Check sheet for the modelled part. Datum: model origin and axes. Units: mm. A direction names the side the tool comes from. Round coordinates to 2 decimals unless told otherwise and drop trailing zeros. Order: outer loops, then holes, each group sorted by start corner. A loop starts at its lowest first (then second) coordinate and runs counter-clockwise, first axis right, second up.
(1) Sectioned sample at D-D, the plane x = 60. Enter the section's corners in (y, z), and give its area (3 significant figures).
(2) Sectioned sample at B-B, the plane z = 17.5. Enter the section's corners in (x, y), and give its area (3 significant figures).
(3) Tool access check on faces 4 (the flat face through (-57.759, 1.568, 41.056)), 5 (the cylindrical face through (-334.68, 1.57, -7.91)), 6 (the flat face through (68.784, 1.568, -0.502)). Record the directions out of +Z, -Z, +X, -X, +Y, -Y that give a thin tool (end or side, any length) a straight path to the whole face; none if there is none.
(4) Sectioned sample at A-A, the plane y = 1.45. Count the separate pieces of the cut face and the enclosed holes in it, and give its area (3 significant figures).
(5) Mould release check, pull along X, two halves, no side actions. Record for faces 1 (the flat face through (5, 0, 20)), 2 (the flat face through (-70.484, 1.568, 0.147)), 3 (the cylindrical face through (226.448, 1.568, 32.697)): released by +X, released by -X, zero draft, split by the parting line, or undercut.
(6) Sectioned sample at C-C, the plane x = 239. Enter the section's corners in (y, z), and give its area (3 significant figures).
(7) Thickness scan on probe 1 along Z at (x, y) = (0, 2.35); probe 2 along Z at (x, y) = (-325, 1.45) (3 decimals); probe 3 along Z at (x, y) = (-229, 2.4). Record the ranges inside material, lowest first.
```python
from build123d import *

# Parameters (mm, degrees)
BOSS_EXTRUDE1_DEPTH = 3.18
SKETCH3_R           = 3.175
SKETCH3_R_2         = 6.35
SKETCH3_R_3         = 1.65
CUT_EXTRUDE1_DEPTH  = 4.18


with BuildPart() as part:
    # Sketch1 → Boss-Extrude1 (new body)
    with BuildSketch(Plane(origin=(0, 0, 0), x_dir=(1, 0, 0), z_dir=(0, 1, 0))):
        with BuildLine():
            Line((-316.883271773, 9.506246519), (-316.457354569, 9.142585196))
            ThreePointArc((-316.457354569, 9.142585196), (-227.815789201, -32.465901654), (-130.352994696, -23.000333716))
            Line((-130.352994696, -23.000333716), (-8.915781366, 23.356130729))
            ThreePointArc((-8.915781366, 23.356130729), (0, 25), (8.915781366, 23.356130729))
            Line((8.915781366, 23.356130729), (130.352994696, -23.000333716))
            ThreePointArc((130.352994696, -23.000333716), (227.815789201, -32.465901654), (316.457354569, 9.142585196))
            Line((316.457354569, 9.142585196), (316.883271773, 9.506246519))
            ThreePointArc((316.883271773, 9.506246519), (334.506246519, 8.116728227), (333.116728227, -9.506246519))
            Line((333.116728227, -9.506246519), (332.690811024, -9.869907842))
            ThreePointArc((332.690811024, -9.869907842), (230.873321689, -60.601151934), (117.157638275, -57.567407196))
            Line((117.157638275, -57.567407196), (0, -25))
            Line((0, -25), (-117.157638275, -57.567407196))
            ThreePointArc((-117.157638275, -57.567407196), (-230.873321689, -60.601151934), (-332.690811024, -9.869907842))
            Line((-332.690811024, -9.869907842), (-333.116728227, -9.506246519))
            ThreePointArc((-333.116728227, -9.506246519), (-334.506246519, 8.116728227), (-316.883271773, 9.506246519))
        make_face()
    extrude(amount=BOSS_EXTRUDE1_DEPTH)

    # Sketch3 → Cut-Extrude1 (cut, through all)
    with BuildSketch(Plane(origin=(0, 3.18, 0), x_dir=(1, 0, 0), z_dir=(0, 1, 0))):
        with Locations((-325, 0)):
            Circle(SKETCH3_R)
        Circle(SKETCH3_R_2)
        with Locations((-260, -45.151120288)):
            Circle(SKETCH3_R_3)
        with Locations((-178.75, -41.327805807)):
            Circle(SKETCH3_R_3)
        with Locations((-81.25, -40.58582431)):
            Circle(SKETCH3_R_3)
        with Locations((81.25, -40.58582431)):
            Circle(SKETCH3_R_3)
        with Locations((178.75, -41.327805807)):
            Circle(SKETCH3_R_3)
        with Locations((260, -45.151120288)):
            Circle(SKETCH3_R_3)
        with Locations((325, 0)):
            Circle(SKETCH3_R)
    extrude(amount=-CUT_EXTRUDE1_DEPTH, mode=Mode.SUBTRACT)


solid = part.part
```
Derived:
1. outline: (0, -3.86) - (3.18, -3.86) - (3.18, 41.68) - (0, 41.68) - close
1. area: 145 mm2
2. outline: (-323.27, 0) - (-275.22, 0) - (-275.22, 3.18) - (-323.27, 3.18) - close; (-115.94, 0) - (115.94, 0) - (115.94, 3.18) - (-115.94, 3.18) - close; (275.22, 0) - (323.27, 0) - (323.27, 3.18) - (275.22, 3.18) - close
2. area: 1,040 mm2
3. face 4: +Z, +Y, -Y
3. face 5: +Y, -Y
3. face 6: -Z, +Y, -Y
4. separate pieces: 1
4. enclosed holes: 9
4. area: 24,000 mm2
5. face 1: zero draft
5. face 2: undercut
5. face 3: undercut
6. outline: (0, 30.18) - (3.18, 30.18) - (3.18, 58.65) - (0, 58.65) - close
6. area: 90.5 mm2
7. probe 1: z = -25 to -6.35, 6.35 to 25
7. probe 2: z = -12.5 to -3.175, 3.175 to 16.16
7. probe 3: z = 32.26 to 61.01
